Autodesk Inventor part; units mm, degrees
ref_plane "YZ Plane" through (0, 0, 0) normal (1, 0, 0) x (0, 1, 0)
ref_plane "XZ Plane" through (0, 0, 0) normal (0, 1, 0) x (-1, 0, 0)
ref_plane "XY Plane" through (0, 0, 0) normal (0, 0, 1) x (1, 0, 0)
sketch "スケッチ1" plane through (0, 0, 0) normal (0, 1, 0) x (-1, 0, 0)
  circle A0 centre (0, 0) radius 12.5
  dimension "d0" = 25
extrude "押し出し1" add sketch "スケッチ1" along normal blind 5
sketch "スケッチ2" plane through (0, 5, 0) normal (0, 1, 0) x (1, 0, 0)
  circle A0 centre (0, 0) radius 12.5
  circle A1 centre (0, 0) radius 1.25
  dimension "d3" = 2.5
extrude "押し出し2" cut sketch "スケッチ2" against normal blind 3 contours A1
sketch "スケッチ3" plane through (0, 0, 0) normal (0, -1, 0) x (1, 0, 0)
  circle A0 centre (0, 0) radius 12.5
  circle A1 centre (0, 0) radius 1.25
  dimension "d6" = 2.5
extrude "押し出し3" add sketch "スケッチ3" along normal blind 3 contours A1
sketch "スケッチ4" plane through (0, 5, 0) normal (0, 1, 0) x (1, 0, 0)
  circle A0 centre (0, 0) radius 12.5
  circle A1 centre (0, 0) radius 17.5
  dimension "d9" = 35
extrude "押し出し4" add sketch "スケッチ4" against normal blind 5
sketch "スケッチ5" plane through (0, 5, 0) normal (0, 1, 0) x (1, 0, 0)
  circle A0 centre (0, 0) radius 17.5
  circle A1 centre (0, 0) radius 1.25
  circle A2 centre (0, 0) radius 22.5
  dimension "d12" = 45
extrude "押し出し5" add sketch "スケッチ5" against normal blind 5 contours A2
properties part number "知能ロボコンシリンダ延長45mm"
The listing builds one solid part. Answer for the finished solid, in the listing's coordinates (mm). A direction names the side the tool comes from. Give positions to 0.01 mm unless a question says otherwise; leave off trailing zeros. Order: outer loops, then holes, each group sorted by start corner. A loop starts at its lowest first (then second) coordinate and runs counter-clockwise, first axis right, second up. Notation, with made-up numbers: (-25, 54) -> (28, 54) arc R17 cw to (28, 71) -> close; hole circle Ø4 at (50.5, 39.25). An arc over 180 degrees is marked (long way). Answer as CSV lines item,"result". Start each with the question number.
Q1. Determine the mould class of faces 1 (the flat face through (0, 5, 5)), 2 (the cylindrical face through (10.382, 2.535, 19.961)), 3 (the cylindrical face through (-0.27, 3.52, 1.22)) for opening direction X: pulls with the +X half, pulls with the -X half, needs draft (parallel to the pull), parting line crosses it, or undercut.
Q2. Find the intervals of material crossed by L1, parallel to X at y = 3.15, z = 0; L2, parallel to Y at x = -19, z = -6.5, in increasing order.
Q3. A cutting plane is placed at B-B (x = 0). Determine the outline of the cut face in (y, z).
Q4. A cutting plane is placed at D-D (y = -2). Determine the outline of the cut face in (x, z), then the cut area to 3 significant figures.
Q5. Which of the six approach directions +Z, -Z, +X, -X, +Y, -Y give full straight-line access (tool end or side, diameter ignored) to faces 4 (the cylindrical face through (-0.27, -1.48, 1.22)), 5 (the flat face through (0, -3, 0)), 6 (the flat face through (0, 2, 0))?
Q6. A cutting plane is placed at C-C (y = 3). Determine the outline of the cut face in (x, z).
Q7. A cutting plane is placed at A-A (z = 0). Determine the outline of the cut face in (x, y), then the cut area to 3 significant figures.
Q8. Given pin 1 (5 mm diameter, centred on x = 7.5, z = -10, fed in from -Y); pin 2 (4 mm diameter, centred on x = -10, y = 1, fed in from +Z); pin 3 (1.5 mm diameter, centred on x = 0, z = 0, fed in from +Y), each flat-ended and moving along its own axis, determine where each tip first touches the part or whether it passes through.
Results found:
1,face 1,"needs draft"
1,face 2,"parting line crosses it"
1,face 3,"undercut"
2,L1,"-22.5 to -1.25, 1.25 to 22.5"
2,L2,"0 to 5"
3,outline,"(-3, -1.25) -> (0, -1.25) -> (0, -22.5) -> (5, -22.5) -> (5, -1.25) -> (2, -1.25) -> (2, 1.25) -> (5, 1.25) -> (5, 22.5) -> (0, 22.5) -> (0, 1.25) -> (-3, 1.25) -> close"
4,outline,"circle Ø2.5 at (0, 0)"
4,area,"4.91 mm2"
5,face 4,"-Y"
5,face 5,"+Z, -Z, +X, -X, -Y"
5,face 6,"+Y"
6,outline,"circle Ø45 at (0, 0); hole circle Ø2.5 at (0, 0)"
7,outline,"(-22.5, 0) -> (-1.25, 0) -> (-1.25, -3) -> (1.25, -3) -> (1.25, 0) -> (22.5, 0) -> (22.5, 5) -> (1.25, 5) -> (1.25, 2) -> (-1.25, 2) -> (-1.25, 5) -> (-22.5, 5) -> close"
7,area,"225 mm2"
8,pin 1,"y = 0"
8,pin 2,"z = 21.03"
8,pin 3,"y = 2"
